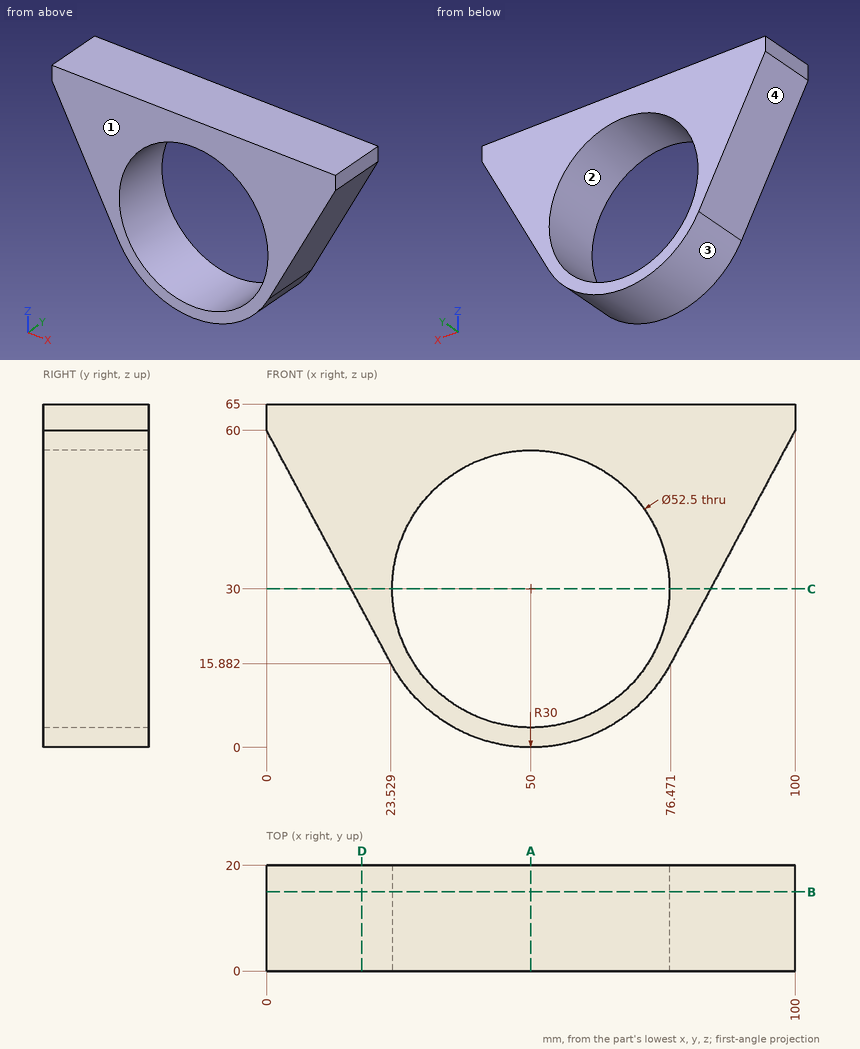
For this review, use the dimensioned drawing (mm, ordinates from the lowest corner) and the shaded views. Give positions to 0.01 mm unless a question says otherwise; leave off trailing zeros. Order: outer loops, then holes, each group sorted by start corner. A loop starts at its lowest first (then second) coordinate and runs counter-clockwise, first axis right, second up. Notation, with made-up numbers: (68, -11) - (100, -11) arc R28 cw to (100, 11) - close; hole circle Ø8 at (29.25, 28). An arc over 180 degrees is marked (long way). Write item = value, one per line. Start each with the question number.
Q1. We need section A-A on x = 50. State the section outline as (y, z) points, plus the area to 3 significant figures.
Q2. To check wall thickness, follow L1, parallel to Z at x = 50, y = 12.25; L2, parallel to X at y = 7.75, z = 30; L3, parallel to Z at x = 64, y = 3.5 (1 decimal). State the ranges of each line that lie inside material, in increasing order. Write a range as from..to.
Q3. Clearance check with flat-ended pins moving along their axes: pin 1 Ø4 at (x, y) = (23.5, 3.5) entering from -Z (1 decimal); pin 2 Ø8 at (y, z) = (8.5, 19.5) entering from -X; pin 3 Ø12 at (x, y) = (24.5, 17.5) entering from -Z. State where each tip first meets the part, or that it passes through.
Q4. We need section B-B on y = 15. State the section outline as (x, z) points.
Q5. We need section D-D on x = 18. State the section outline as (y, z) points.
Q6. We need section C-C on z = 30. State the section outline as (x, y) points, plus the area to 3 significant figures.
Q7. Mouldability with a two-part tool opening along X and no side actions: class the marked faces 1, 2, 3 and 4 as released by +X, released by -X, zero draft, split by the parting line, or undercut.
Working result:
q1.outline = (0, 0) - (20, 0) - (20, 3.75) - (0, 3.75) - close; (0, 56.25) - (20, 56.25) - (20, 65) - (0, 65) - close
q1.area = 250 mm²
q2.L1 = 0..3.75, 56.25..65
q2.L2 = 16..23.75, 76.25..84
q2.L3 = 3.5..7.8, 52.2..65
q3.pin_1 = 12.7
q3.pin_2 = 19.47
q3.pin_3 = 7.2
q4.outline = (0, 60) - (23.53, 15.88) arc R30 ccw to (76.47, 15.88) - (100, 60) - (100, 65) - (0, 65) - close; hole circle Ø52.5 at (50, 30)
q5.outline = (0, 26.25) - (20, 26.25) - (20, 65) - (0, 65) - close
q6.outline = (16, 0) - (23.75, 0) - (23.75, 20) - (16, 20) - close; (76.25, 0) - (84, 0) - (84, 20) - (76.25, 20) - close
q6.area = 310 mm²
q7.face_1 = zero draft
q7.face_2 = undercut
q7.face_3 = split by the parting line
q7.face_4 = released by -X
